```python
from build123d import *

# Parameters (mm, degrees)
SKETCH1_W                    = 189.8572
SKETCH1_H                    = 175.514
BASE_FLANGE1_DEPTH           = 2.3
EDGE_FLANGE4_STRIP_W         = 10.8256
EDGE_FLANGE4_STRIP_H         = 2.3
EDGE_FLANGE4_STRIP_CUT_DEPTH = 189.8572
EDGE_FLANGE4_DEPTH           = 189.8572
CUT_EXTRUDE1_DEPTH           = 144.797004807
CUT_EXTRUDE5_REACH           = 150.616
SKETCH41_R                   = 2.4765
CUT_EXTRUDE6_REACH           = 137.965
SKETCH42_R                   = 2.413
SKETCH42_R_2                 = 2.4765


# Sheet-metal steps are written as plain solids
with BuildPart() as part:
    # Sketch1 → Base-Flange1 (new body)
    with BuildSketch(Plane(origin=(0, 0, 0), x_dir=(1, 0, 0), z_dir=(0, 1, 0))):
        with Locations((11.4698, 7.08)):
            Rectangle(SKETCH1_W, SKETCH1_H)
    extrude(amount=-BASE_FLANGE1_DEPTH)

    # Edge-Flange4 strip (across the edge) → Edge-Flange4 strip cut (cut)
    with BuildSketch(Plane(origin=(-83.4588, 0, 80.677), x_dir=(0, 0, -1), z_dir=(1, 0, 0))):
        with Locations((-4.6, -1.15)):
            Rectangle(EDGE_FLANGE4_STRIP_W, EDGE_FLANGE4_STRIP_H)
    extrude(amount=EDGE_FLANGE4_STRIP_CUT_DEPTH, mode=Mode.SUBTRACT)

    # Edge-Flange4 section (across the edge) → Edge-Flange4 (add)
    with BuildSketch(Plane(origin=(-83.4588, 0, 80.677), x_dir=(0, 0, -1), z_dir=(1, 0, 0))):
        with BuildLine():
            Line((-2.3, 0.8128), (-2.3, 16.75))
            Line((-2.3, 16.75), (0, 16.75))
            Line((0, 16.75), (0, 0.8128))
            ThreePointArc((0, 0.8128), (0.238063608, 0.238063608), (0.8128, 0))
            Line((0.8128, 0), (0.8128, -2.3))
            ThreePointArc((0.8128, -2.3), (-1.388281988, -1.388281988), (-2.3, 0.8128))
        make_face()
    extrude(amount=EDGE_FLANGE4_DEPTH)

    # Sketch36 → Cut-Extrude1 (cut, through all)
    with BuildSketch(Plane.XZ.offset(2.3)):
        Polygon((19.845566889, -21.7218), (-83.4588, -21.7218), (-83.4588, -94.837), (106.3984, -94.837), (106.3984, 50.90465034), align=None)
    extrude(amount=-CUT_EXTRUDE1_DEPTH, mode=Mode.SUBTRACT)

    # Sketch41 → Cut-Extrude5 (cut, up to next)
    with BuildSketch(Plane(origin=(0, 0, 80.677), x_dir=(-1, 0, 0), z_dir=(0, 0, -1)), mode=Mode.PRIVATE) as cut_extrude5_sk1:
        with Locations(Location((64.7302, 8.7814, 0), (0, 0, 90))):
            Circle(SKETCH41_R)
    cut_extrude5_tool1 = extrude(cut_extrude5_sk1.sketch, amount=-CUT_EXTRUDE5_REACH, mode=Mode.PRIVATE) & part.part
    # Sketch41 → Cut-Extrude5 (cut, up to next)
    with BuildSketch(Plane(origin=(0, 0, 80.677), x_dir=(-1, 0, 0), z_dir=(0, 0, -1)), mode=Mode.PRIVATE) as cut_extrude5_sk2:
        with Locations(Location((39.3302, 8.7814, 0), (0, 0, 90))):
            Circle(SKETCH41_R)
    cut_extrude5_tool2 = extrude(cut_extrude5_sk2.sketch, amount=-CUT_EXTRUDE5_REACH, mode=Mode.PRIVATE) & part.part
    # Sketch41 → Cut-Extrude5 (cut, up to next)
    with BuildSketch(Plane(origin=(0, 0, 80.677), x_dir=(-1, 0, 0), z_dir=(0, 0, -1)), mode=Mode.PRIVATE) as cut_extrude5_sk3:
        with Locations(Location((13.9302, 8.7814, 0), (0, 0, 90))):
            Circle(SKETCH41_R)
    cut_extrude5_tool3 = extrude(cut_extrude5_sk3.sketch, amount=-CUT_EXTRUDE5_REACH, mode=Mode.PRIVATE) & part.part
    # Sketch41 → Cut-Extrude5 (cut, up to next)
    with BuildSketch(Plane(origin=(0, 0, 80.677), x_dir=(-1, 0, 0), z_dir=(0, 0, -1)), mode=Mode.PRIVATE) as cut_extrude5_sk4:
        with Locations(Location((-11.4698, 8.7814, 0), (0, 0, 90))):
            Circle(SKETCH41_R)
    cut_extrude5_tool4 = extrude(cut_extrude5_sk4.sketch, amount=-CUT_EXTRUDE5_REACH, mode=Mode.PRIVATE) & part.part
    # Sketch41 → Cut-Extrude5 (cut, up to next)
    with BuildSketch(Plane(origin=(0, 0, 80.677), x_dir=(-1, 0, 0), z_dir=(0, 0, -1)), mode=Mode.PRIVATE) as cut_extrude5_sk5:
        with Locations(Location((-36.8698, 8.7814, 0), (0, 0, 90))):
            Circle(SKETCH41_R)
    cut_extrude5_tool5 = extrude(cut_extrude5_sk5.sketch, amount=-CUT_EXTRUDE5_REACH, mode=Mode.PRIVATE) & part.part
    # Sketch41 → Cut-Extrude5 (cut, up to next)
    with BuildSketch(Plane(origin=(0, 0, 80.677), x_dir=(-1, 0, 0), z_dir=(0, 0, -1)), mode=Mode.PRIVATE) as cut_extrude5_sk6:
        with Locations(Location((-62.2698, 8.7814, 0), (0, 0, 90))):
            Circle(SKETCH41_R)
    cut_extrude5_tool6 = extrude(cut_extrude5_sk6.sketch, amount=-CUT_EXTRUDE5_REACH, mode=Mode.PRIVATE) & part.part
    # Sketch41 → Cut-Extrude5 (cut, up to next)
    with BuildSketch(Plane(origin=(0, 0, 80.677), x_dir=(-1, 0, 0), z_dir=(0, 0, -1)), mode=Mode.PRIVATE) as cut_extrude5_sk7:
        with Locations(Location((-87.6698, 8.7814, 0), (0, 0, 90))):
            Circle(SKETCH41_R)
    cut_extrude5_tool7 = extrude(cut_extrude5_sk7.sketch, amount=-CUT_EXTRUDE5_REACH, mode=Mode.PRIVATE) & part.part
    add(cut_extrude5_tool1.solids().sort_by_distance((-64.7302, 8.7814, 80.677))[0], mode=Mode.SUBTRACT)
    add(cut_extrude5_tool2.solids().sort_by_distance((-39.3302, 8.7814, 80.677))[0], mode=Mode.SUBTRACT)
    add(cut_extrude5_tool3.solids().sort_by_distance((-13.9302, 8.7814, 80.677))[0], mode=Mode.SUBTRACT)
    add(cut_extrude5_tool4.solids().sort_by_distance((11.4698, 8.7814, 80.677))[0], mode=Mode.SUBTRACT)
    add(cut_extrude5_tool5.solids().sort_by_distance((36.8698, 8.7814, 80.677))[0], mode=Mode.SUBTRACT)
    add(cut_extrude5_tool6.solids().sort_by_distance((62.2698, 8.7814, 80.677))[0], mode=Mode.SUBTRACT)
    add(cut_extrude5_tool7.solids().sort_by_distance((87.6698, 8.7814, 80.677))[0], mode=Mode.SUBTRACT)

    # Sketch42 → Cut-Extrude6 (cut, up to next)
    with BuildSketch(Plane(origin=(0, 0, 0), x_dir=(1, 0, 0), z_dir=(0, 1, 0)), mode=Mode.PRIVATE) as cut_extrude6_sk1:
        with Locations(Location((-75.4832, 8.3218, 0), (0, 0, 270))):
            Circle(SKETCH42_R)
    cut_extrude6_tool1 = extrude(cut_extrude6_sk1.sketch, amount=-CUT_EXTRUDE6_REACH, mode=Mode.PRIVATE) & part.part
    # Sketch42 → Cut-Extrude6 (cut, up to next)
    with BuildSketch(Plane(origin=(0, 0, 0), x_dir=(1, 0, 0), z_dir=(0, 1, 0)), mode=Mode.PRIVATE) as cut_extrude6_sk2:
        with Locations(Location((-75.4832, -17.0782, 0), (0, 0, 270))):
            Circle(SKETCH42_R)
    cut_extrude6_tool2 = extrude(cut_extrude6_sk2.sketch, amount=-CUT_EXTRUDE6_REACH, mode=Mode.PRIVATE) & part.part
    # Sketch42 → Cut-Extrude6 (cut, up to next)
    with BuildSketch(Plane(origin=(0, 0, 0), x_dir=(1, 0, 0), z_dir=(0, 1, 0)), mode=Mode.PRIVATE) as cut_extrude6_sk3:
        with Locations(Location((-75.4832, -42.4782, 0), (0, 0, 270))):
            Circle(SKETCH42_R)
    cut_extrude6_tool3 = extrude(cut_extrude6_sk3.sketch, amount=-CUT_EXTRUDE6_REACH, mode=Mode.PRIVATE) & part.part
    # Sketch42 → Cut-Extrude6 (cut, up to next)
    with BuildSketch(Plane(origin=(0, 0, 0), x_dir=(1, 0, 0), z_dir=(0, 1, 0)), mode=Mode.PRIVATE) as cut_extrude6_sk4:
        with Locations(Location((-75.4832, -67.8782, 0), (0, 0, 270))):
            Circle(SKETCH42_R)
    cut_extrude6_tool4 = extrude(cut_extrude6_sk4.sketch, amount=-CUT_EXTRUDE6_REACH, mode=Mode.PRIVATE) & part.part
    # Sketch42 → Cut-Extrude6 (cut, up to next)
    with BuildSketch(Plane(origin=(0, 0, 0), x_dir=(1, 0, 0), z_dir=(0, 1, 0)), mode=Mode.PRIVATE) as cut_extrude6_sk5:
        with Locations(Location((98.4228, -59.3042, 0), (0, 0, 270))):
            Circle(SKETCH42_R_2)
    cut_extrude6_tool5 = extrude(cut_extrude6_sk5.sketch, amount=-CUT_EXTRUDE6_REACH, mode=Mode.PRIVATE) & part.part
    # Sketch42 → Cut-Extrude6 (cut, up to next)
    with BuildSketch(Plane(origin=(0, 0, 0), x_dir=(1, 0, 0), z_dir=(0, 1, 0)), mode=Mode.PRIVATE) as cut_extrude6_sk6:
        with Locations(Location((98.4228, -72.0042, 0), (0, 0, 270))):
            Circle(SKETCH42_R_2)
    cut_extrude6_tool6 = extrude(cut_extrude6_sk6.sketch, amount=-CUT_EXTRUDE6_REACH, mode=Mode.PRIVATE) & part.part
    add(cut_extrude6_tool1.solids().sort_by_distance((-75.4832, 0, -8.3218))[0], mode=Mode.SUBTRACT)
    add(cut_extrude6_tool2.solids().sort_by_distance((-75.4832, 0, 17.0782))[0], mode=Mode.SUBTRACT)
    add(cut_extrude6_tool3.solids().sort_by_distance((-75.4832, 0, 42.4782))[0], mode=Mode.SUBTRACT)
    add(cut_extrude6_tool4.solids().sort_by_distance((-75.4832, 0, 67.8782))[0], mode=Mode.SUBTRACT)
    add(cut_extrude6_tool5.solids().sort_by_distance((98.4228, 0, 59.3042))[0], mode=Mode.SUBTRACT)
    add(cut_extrude6_tool6.solids().sort_by_distance((98.4228, 0, 72.0042))[0], mode=Mode.SUBTRACT)


solid = part.part
```
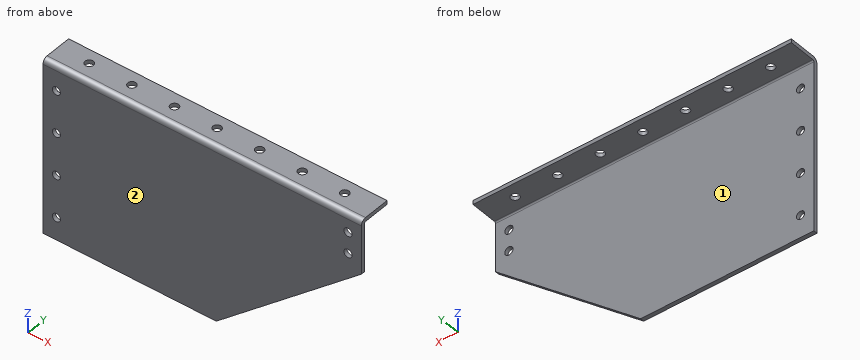
Geometry: final body of the model. Coordinates: model frame, mm. Face numbers are marked on the shaded views. A direction names the side the tool comes from. Give positions to 0.01 mm unless a question says otherwise; leave off trailing zeros. Write each loop counter-clockwise with the first axis right and the second up, starting at its lowest first coordinate (ties: lowest second). Pieces come first, ordered by that corner, then holes.
1. Line query: probe 1 along Y at (x, z) = (41, 25.5); probe 2 along Z at (x, y) = (-64, 1). Output: solid intervals per line, ascending.
2. Section query D-D, the plane z = 16.5. Return loops of the section in (x, y).
3. Section query B-B, the plane z = 59. Return loops of the section in (x, y), then the cut area to 3 significant figures.
4. Section query C-C, the plane x = 16. Return loops of the section in (y, z).
5. Section query A-A, the plane y = 8.5. Count the separate pieces of the cut face and the enclosed holes in it, then the cut area to 3 significant figures.
6. Pin query (flat end, axial travel): P1, Ø7.5, axis at x = -75.48, z = -8.32, coming from the +Y side; P2, Ø6.5, axis at x = -39.33, y = 8.78, coming from the -Z side; P3, Ø10, axis at y = -0.5, z = 5.5, coming from the +X side. Return the tip coordinate at first contact, or that it passes through.
7. Reachability of the marked faces 1 and 2 from +Z, -Z, +X, -X, +Y, -Y: full face, straight path, thin tool, end or side. Return the list, or none.
Computed:
1. probe 1: y = -2.3 to 0
1. probe 2: z = 80.68 to 82.98
2. outline: (-83.46, -2.3) - (-77.83, -2.3) - (-77.83, 0) - (-83.46, 0) - close; (-73.14, -2.3) - (65.4, -2.3) - (65.4, 0) - (-73.14, 0) - close
3. outline: (-83.46, -2.3) - (95.97, -2.3) - (95.97, 0) - (-83.46, 0) - close; (100.88, -2.3) - (106.4, -2.3) - (106.4, 0) - (100.88, 0) - close
3. area: 425 mm2
4. outline: (-2.3, -21.72) - (0, -21.72) - (0, 79.86) arc R0.81 cw to (0.81, 80.68) - (16.75, 80.68) - (16.75, 82.98) - (0.81, 82.98) arc R3.11 ccw to (-2.3, 79.86) - close
5. separate pieces: 8
5. enclosed holes: 0
5. area: 357 mm2
6. P1: stops at y = 0
6. P2: stops at z = 80.68
6. P3: stops at x = 58.25
7. face 1: -Z, +X, -X, +Y
7. face 2: +Z, -Z, +X, -X, -Y
